Source: three-view drawing plus pictorial views. Frame: mm from the lowest corner of the part. A direction names the side the tool comes from. Coordinates: 2 decimals unless noted, no trailing zeros. Write each loop counter-clockwise with the first axis right and the second up, starting at its lowest first coordinate (ties: lowest second). Pieces come first, ordered by that corner, then holes. Notation, with made-up numbers: (65, -38) - (74, -38) arc R15 cw to (74, -33) - close; hole circle Ø6 at (-32.75, 68.25). An arc over 180 degrees is marked (long way). Put each result on its own line as item: value. Start each with the question number.
1. Cut plane A-A, the plane x = 2.5. Return loops of the section in (y, z) (3 decimals), and give its area (3 significant figures).
2. Pin query (flat end, axial travel): pin 1 (1.2 mm diameter, centred on x = 2.5, y = 2.5, fed in from +Z) (3 decimals); pin 2 (3 mm diameter, centred on x = 4, z = 6, fed in from +Y). Return the tip coordinate at first contact, or that it passes through.
3. Cut plane B-B, the plane z = 6.5. Return loops of the section in (x, y), and give its area (3 significant figures).
4. Access query for the marked faces 4 and 5. Directions: +Z, -Z, +X, -X, +Y, -Y. A direction counts if a zero-diameter tool reaches every point of the face in a straight line with its end or side. Return the directions, or none.
5. Pull-direction query (X, two-part tool) for the marked faces 1, 2 and 3; classes: released by +X, released by -X, zero draft, split by the parting line, or undercut.
6. Line query: line 1 (Z direction, x = 4.25, y = 3.15); line 2 (Y direction, x = 2.5, z = 4); line 3 (X direction, y = 3.25, z = 6). Output: solid intervals per line, ascending.
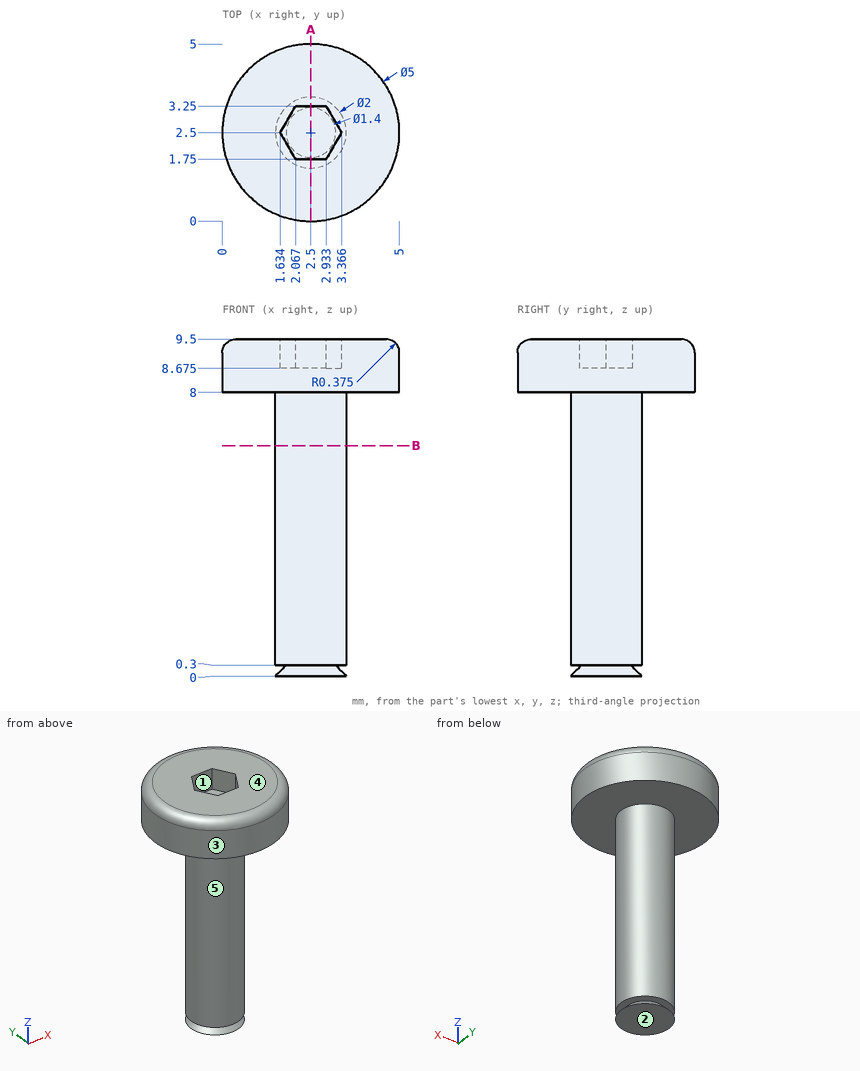
Report:
1. outline: (0, 8) - (1.5, 8) - (1.5, 0.3) - (1.8, 0.3) - (1.5, 0) - (3.5, 0) - (3.2, 0.3) - (3.5, 0.3) - (3.5, 8) - (5, 8) - (5, 9.125) arc R0.375 ccw to (4.625, 9.5) - (3.25, 9.5) - (3.25, 8.675) - (1.75, 8.675) - (1.75, 9.5) - (0.375, 9.5) arc R0.375 ccw to (0, 9.125) - close
1. area: 22.1 mm^2
2. pin 1: stops at z = 8.675
2. pin 2: stops at y = 3.5
3. outline: circle Ø2 at (2.5, 2.5)
3. area: 3.14 mm^2
4. face 4: +Z, +X, -X, +Y, -Y
4. face 5: -Z
5. face 1: undercut
5. face 2: zero draft
5. face 3: split by the parting line
6. line 1: z = 8 to 9.5
6. line 2: y = 1.5 to 3.5
6. line 3: x = 1.84 to 3.16
